Could you check a few things on this model? Use its own coordinates, in mm. Face numbers are marked on the shaded views. A direction names the side the tool comes from. Coordinates: 2 decimals unless noted, no trailing zeros. Order: outer loops, then holes, each group sorted by start corner. A loop starts at its lowest first (then second) coordinate and runs counter-clockwise, first axis right, second up. Notation, with made-up numbers: M 45,-23 L 52,-23 A17 ccw 52,-12 Z; hole C 10.25,-17.5 d4. An arc over 180 degrees is marked long. Put each result on its own line as item: value. Start each with the question number.
Autodesk Inventor part; units mm, degrees
ref_plane "YZ Plane" through (0, 0, 0) normal (1, 0, 0) x (0, 1, 0)
ref_plane "XZ Plane" through (0, 0, 0) normal (0, 1, 0) x (-1, 0, 0)
ref_plane "XY Plane" through (0, 0, 0) normal (0, 0, 1) x (1, 0, 0)
sketch "スケッチ1" plane through (0, 0, 0) normal (0, 1, 0) x (-1, 0, 0)
  line L0 (0, 0) -> (-5, 0)
  line L1 (-5, 0) -> (-5, 2.8)
  line L2 (-5, 2.8) -> (-3, 2.8)
  line L3 (-3, 2.8) -> (-3, 7.3)
  line L4 (-3, 7.3) -> (-2, 7.3)
  line L5 (-2, 7.3) -> (-2, 11.87)
  line L6 (-1.57, 12.3) -> (0, 12.3)
  line L7 (0, 12.3) -> (0, 0)
  line L8 (-1.57, 12.3) -> (-2, 11.87)
  point P0 (-2, 12.3)
  dimension "d0" = 5
  dimension "d1" = 4.5
  dimension "d2" = 2.8
  dimension "d3" = 0.43
  dimension "d4" = 0.43
  dimension "d5" = 4
  dimension "d6" = 10
  dimension "d7" = 6
revolve "回転1" add sketch "スケッチ1" angle 360 about axis through (0, 0, 12.3) along (0, 0, -1)
thread "ねじ1"
sketch "スケッチ2" plane through (0, 0, 0) normal (0, 0, -1) x (-1, 0, 0)
  line L0 (0, -1.4434) -> (-1.25, -0.7217)
  line L1 (-1.25, -0.7217) -> (-1.25, 0.7217)
  line L2 (-1.25, 0.7217) -> (0, 1.4434)
  line L3 (0, 1.4434) -> (1.25, 0.7217)
  line L4 (1.25, 0.7217) -> (1.25, -0.7217)
  line L5 (1.25, -0.7217) -> (0, -1.4434)
  point P0 (0, 0)
  point P1 (0, 0)
  dimension "d11" = 2.5
extrude "押し出し1" cut sketch "スケッチ2" against normal blind 1.5
properties part number "DBTS4-4.5-5-LTC" material "ステンレス鋼 AISI 304"
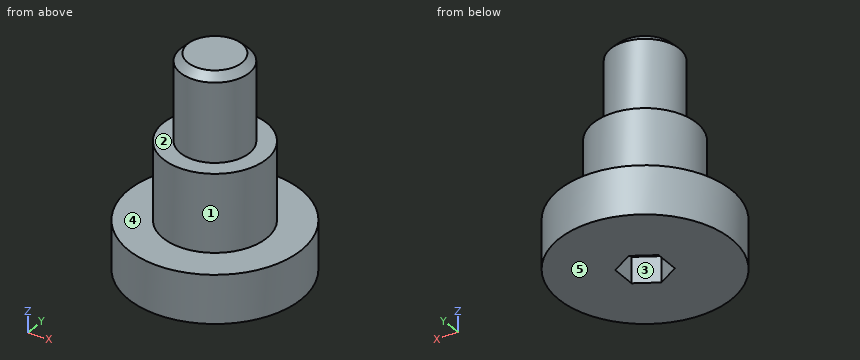
Item 1: If we section it at C-C on x = -4: Write out the boundary of the cut face in (y, z).
Item 2: For the marked faces 4 and 5, which set-ups out of +Z, -Z, +X, -X, +Y, -Y let a thin tool reach every point of the face, with its end or its side?
Item 3: If we section it at B-B on z = 5.5: Write out the boundary of the cut face in (x, y), then the cut area to 3 significant figures.
Item 4: If we section it at D-D on y = 3.25: Write out the boundary of the cut face in (x, z).
Item 5: If we mould it in two halves opening along X, with no side actions, what happens to the marked faces 1, 2 and 3? For each: released by +X, released by -X, zero draft, split by the parting line, or undercut.
Item 6: If we section it at A-A on y = 0: Write out the boundary of the cut face in (x, z).
Item 7: I need wall thicknesses on probe 1 along Z at (x, y) = (0.5, -1); probe 2 along Z at (x, y) = (-4.5, -0.5); probe 3 along X at (y, z) = (0, 11.25). Which ranges of each line are inside material? Lowest first, please.
Item 8: For pin 1 Ø6 at (y, z) = (1, 9) entering from -X; pin 2 Ø5 at (x, z) = (-1, 6) entering from +Y; pin 3 Ø0.8 at (x, y) = (-0.5, -0.5) entering from -Z, each with a flat end and sliding along its axis, tell me the tip position at first contact or that it passes through.
Geometry check:
1. outline: M -3,0 L 3,0 L 3,2.8 L -3,2.8 Z
2. face 4: +Z
2. face 5: -Z, +X, -X, +Y, -Y
3. outline: C 0,0 d6
3. area: 28.3 mm²
4. outline: M -3.8,0 L 3.8,0 L 3.8,2.8 L -3.8,2.8 Z
5. face 1: split by the parting line
5. face 2: zero draft
5. face 3: undercut
6. outline: M -5,0 L -1.25,0 L -1.25,1.5 L 1.25,1.5 L 1.25,0 L 5,0 L 5,2.8 L 3,2.8 L 3,7.3 L 2,7.3 L 2,11.87 L 1.57,12.3 L -1.57,12.3 L -2,11.87 L -2,7.3 L -3,7.3 L -3,2.8 L -5,2.8 Z
7. probe 1: z = 1.5 to 12.3
7. probe 2: z = 0 to 2.8
7. probe 3: x = -2 to 2
8. pin 1: stops at x = -3
8. pin 2: stops at y = 3
8. pin 3: stops at z = 1.5
